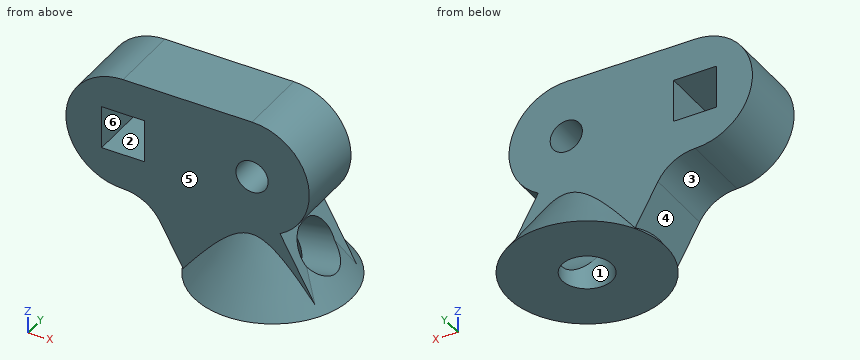
```python
from build123d import *

# Parameters (mm, degrees)
SKETCH023_R       = 2.25
SKETCH023_W       = 6
SKETCH023_H       = 6
PAD017_DEPTH      = 5
CYLINDER060_R     = 3.5
CYLINDER060_DEPTH = 5
CYLINDER061_R     = 3.5
CYLINDER061_DEPTH = 10


with BuildPart() as part:
    # Sketch023 → Pad017 (new body, symmetric)
    with BuildSketch(Plane.XZ):
        with BuildLine():
            Line((-9.5, 0), (-12.806838, 5.911152))
            ThreePointArc((-12.806838, 5.911152), (-15.000053, 8.152854), (-18.024663, 8.981801))
            ThreePointArc((-18, 24.981763), (-25.99999, 16.994094), (-18.024663, 8.981801))
            Line((0, 24.981763), (-18, 24.981763))
            ThreePointArc((3.905763, 10), (7.741256, 18.999918), (0, 24.981763))
            Line((3.905763, 10), (9.5, 0))
            Line((-9.5, 0), (9.5, 0))
        make_face()
        with Locations((0, 16.981763)):
            Circle(SKETCH023_R, mode=Mode.SUBTRACT)
        with Locations((-18, 16.981763)):
            Rectangle(SKETCH023_W, SKETCH023_H, mode=Mode.SUBTRACT)
    extrude(amount=PAD017_DEPTH, both=True)

    # Cone004 → Cone004 (revolve)
    with BuildSketch(Plane.XZ):
        Polygon((0, 0), (11, 0), (4, 10), (0, 10), align=None)
    revolve(axis=Axis((0, 0, 0), (0, 0, 1)))

    # Cylinder060 → Cylinder060 (cut)
    with BuildSketch(Plane.XY):
        Circle(CYLINDER060_R)
    extrude(amount=CYLINDER060_DEPTH, mode=Mode.SUBTRACT)

    # Cylinder061 → Cylinder061 (cut)
    with BuildSketch(Plane(origin=(0, 0, 5), x_dir=(0, 1, 0), z_dir=(0.984808, 0, 0.173648))):
        Circle(CYLINDER061_R)
    extrude(amount=CYLINDER061_DEPTH, mode=Mode.SUBTRACT)

    # Sphere001 → Sphere001 (revolve, cut)
    with BuildSketch(Plane(origin=(0, 0, 5), x_dir=(1, 0, 0), z_dir=(0, -1, 0))):
        with BuildLine():
            ThreePointArc((0, -3.5), (3.5, 0), (0, 3.5))
            Line((0, 3.5), (0, -3.5))
        make_face()
    revolve(axis=Axis((0, 0, 5), (0, 0, 1)), mode=Mode.SUBTRACT)


with BuildPart() as part_1:
    # Body029 placement: moved
    add(part.part.moved(Location((0, 0, 35))))


solid = part_1.part
```
Source: CAD feature listing. Evaluate the final solid. Frame: model axes, mm. Face numbers are marked on the shaded views. A direction names the side the tool comes from. Coordinates: 2 decimals unless noted, no trailing zeros. Loops run counter-clockwise (first coordinate to the right, second up) from the corner with the lowest first, then second, coordinate; pieces in that order, holes last. Notation, with made-up numbers: M 79,41.25 L 111,41.25 A27 ccw 111,59.25 Z; hole C 11.5,18 d2. An arc over 180 degrees is marked long. Put each result on its own line as item: value. Start each with the question number.
1) Pull-direction query (X, two-part tool) for the marked faces 4, 5 and 6; classes: pulls with the +X half, pulls with the -X half, needs draft (parallel to the pull), parting line crosses it, or undercut.
2) Cut plane C-C on y = -4.5. Give the number of separate pieces and of enclosed holes in the cut face, then the cut area to 3 significant figures.
3) Contact query for flat-ended pins moving along their axis: pin 1 Ø1.5 at (y, z) = (4.5, 48) entering from -X; pin 2 Ø1.8 at (x, y) = (-17, 2) entering from -Z; pin 3 Ø6 at (y, z) = (-3.5, 39.5) entering from -X. Output: stop coordinate, or through.
4) Reachability of the marked faces 1, 2 and 3 from +Z, -Z, +X, -X, +Y, -Y: full face, straight path, thin tool, end or side. Return the list, or none.
5) Cut plane B-B on z = 47.5. Return the cut outline in (x, y), then the cut area to 3 significant figures.
6) Ray query, L1, parallel to Y at x = 3, z = 48.5; L2, parallel to Y at x = -1.5, z = 40.25; L3, parallel to X at y = -4.75, z = 50.5. Return the intervals inside material, ascending. Write a range as from..to.
7) Cut plane A-A on y = 0. Return the cut outline in (x, z).
The answers:
1. face 4: pulls with the -X half
1. face 5: needs draft
1. face 6: undercut
2. separate pieces: 1
2. enclosed holes: 2
2. area: 612 mm²
3. pin 1: stops at x = -25.32
3. pin 2: stops at z = 43.66
3. pin 3: stops at x = -14.1
4. face 1: -Z
4. face 2: +Y, -Y
4. face 3: -Z, -X, +Y, -Y
5. outline: M -24.63,-5 L 6.63,-5 L 6.63,5 L -24.63,5 Z
5. area: 313 mm²
6. L1: y = -5..5
6. L2: y = -7.17..-3.15, 3.15..7.17
6. L3: x = -25.86..-21, -15..-1.69, 1.69..7.86
7. outline: M -18.02,43.98 A6 cw -12.81,40.91 L -10.17,36.19 L -11,35 L -3.5,35 L -3.5,40 A3.5 cw -0.61,43.45 L 4.46,44.34 L 4,45 L 3.91,45 A8 ccw 0,59.98 L -18,59.98 A8 ccw Z; M 3.5,35 L 11,35 L 8.89,38.01 L 3.5,37.06 Z; hole M -21,48.98 L -15,48.98 L -15,54.98 L -21,54.98 Z; hole C 0,51.98 d4.5
